Geometry check sheet. Reference: the model listing, model coordinates, mm. A direction names the side the tool comes from. Give positions to 0.01 mm unless a question says otherwise; leave off trailing zeros. Loops run counter-clockwise (first coordinate to the right, second up) from the corner with the lowest first, then second, coordinate; pieces in that order, holes last. Notation, with made-up numbers: (38, 20) -> (87, 20) arc R18 ccw to (87, 28) -> close; hole circle Ø9 at (59.5, 49.5). An arc over 180 degrees is marked (long way). One line per item, written item: value. Start each with the question number.
(1) Sectioned sample at A-A, the plane z = 0. Record the cut outline in (x, y) (3 decimals), then the cut area to 3 significant figures.
(2) Gauge pin test, flat ends, axial feed: pin 1 Ø4 at (y, z) = (6, -8.5) entering from +X; pin 2 Ø1.5 at (y, z) = (6.5, -4) entering from -X; pin 3 Ø5 at (x, y) = (10, 14.5) entering from +Z. Record the tip position at first contact, or that the pin passes through.
(3) Tool access check on faces 1 (the face through (0, 4, -2)), 2 (the face through (0, 17, 0)), 3 (the face through (2, 0, -10)). Record the directions out of +Z, -Z, +X, -X, +Y, -Y that give a thin tool (end or side, any length) a straight path to the whole face; none if there is none.
(4) Scan lines: line 1 along Z through (x, y) = (0, 17.4); line 2 along X through (y, z) = (10.25, 0); line 3 along Z through (x, y) = (2.5, 6.5). Record each from-to range of solid material in increasing order. Write a range as from..to.
(5) Sectioned sample at C-C, the plane x = 0. Record the cut outline in (y, z) (3 decimals), then the cut area to 3 significant figures.
(6) Sectioned sample at D-D, the plane x = 7.25. Record the cut outline in (y, z).
(7) Draft check along Z on faces 4 (the face through (-2.17, 3.94, -9.76)), 5 (the face through (2, 18, -10)), 6 (the face through (7.123, 8.874, -11.172)). Enter one of: pulls with the +Z half, pulls with the -Z half, needs draft (parallel to the pull), parting line crosses it, or undercut.
(8) Sectioned sample at B-B, the plane y = 3. Record the cut outline in (x, z), then the cut area to 3 significant figures.
from build123d import *

# Parameters (mm, degrees)
SKETCH1_R           = 13.25
BOSS_EXTRUDE1_DEPTH = 35
SKETCH7_R           = 10
CUT_EXTRUDE4_DEPTH  = 8
SKETCH10_R          = 3.485
BOSS_EXTRUDE3_DEPTH = 4
CUT_EXTRUDE5_DEPTH  = 8.75
SKETCH13_R          = 10
CUT_EXTRUDE6_DEPTH  = 18
SKETCH14_R          = 13.25
CUT_EXTRUDE7_DEPTH  = 17


with BuildPart() as part:
    # Sketch1 → Boss-Extrude1 (new body)
    with BuildSketch(Plane(origin=(0, 0, 0), x_dir=(1, 0, 0), z_dir=(0, 1, 0))):
        Circle(SKETCH1_R)
    extrude(amount=BOSS_EXTRUDE1_DEPTH)

    # Sketch7 → Cut-Extrude4 (cut)
    with BuildSketch(Plane.XZ):
        Circle(SKETCH7_R)
    extrude(amount=-CUT_EXTRUDE4_DEPTH, mode=Mode.SUBTRACT)

    # Sketch10 → Boss-Extrude3 (add)
    with BuildSketch(Plane.XZ.offset(-8)):
        Circle(SKETCH10_R)
    extrude(amount=BOSS_EXTRUDE3_DEPTH)

    # Sketch11 → Cut-Extrude5 (cut)
    with BuildSketch(Plane.XZ.offset(-4)):
        with BuildLine():
            Line((1.123990489, -1.161812868), (-1.123990489, -1.161812868))
            ThreePointArc((-1.123990489, -1.161812868), (0, 1.616528304), (1.123990489, -1.161812868))
        make_face()
    extrude(amount=-CUT_EXTRUDE5_DEPTH, mode=Mode.SUBTRACT)

    # Sketch13 → Cut-Extrude6 (cut)
    with BuildSketch(Plane(origin=(0, 35, 0), x_dir=(1, 0, 0), z_dir=(0, 1, 0))):
        Circle(SKETCH13_R)
    extrude(amount=-CUT_EXTRUDE6_DEPTH, mode=Mode.SUBTRACT)

    # Sketch14 → Cut-Extrude7 (cut)
    with BuildSketch(Plane(origin=(0, 35, 0), x_dir=(1, 0, 0), z_dir=(0, 1, 0))):
        Circle(SKETCH14_R)
    extrude(amount=-CUT_EXTRUDE7_DEPTH, mode=Mode.SUBTRACT)


solid = part.part
Calculated:
1. outline: (-13.25, 0) -> (-10, 0) -> (-10, 8) -> (-3.485, 8) -> (-3.485, 4) -> (-1.617, 4) -> (-1.617, 12.75) -> (1.617, 12.75) -> (1.617, 4) -> (3.485, 4) -> (3.485, 8) -> (10, 8) -> (10, 0) -> (13.25, 0) -> (13.25, 18) -> (10, 18) -> (10, 17) -> (-10, 17) -> (-10, 18) -> (-13.25, 18) -> close
1. area: 297 mm2
2. pin 1: stops at x = 11.55
2. pin 2: stops at x = -12.85
2. pin 3: stops at z = 10.92
3. face 1: -Y
3. face 2: +Y
3. face 3: +Z, -Z, +X, -X, -Y
4. line 1: z = -13.25..-10, 10..13.25
4. line 2: x = -13.25..-1.62, 1.62..13.25
4. line 3: z = -13.01..-9.68, -2.43..2.43, 9.68..13.01
5. outline: (0, -13.25) -> (18, -13.25) -> (18, -10) -> (17, -10) -> (17, 10) -> (18, 10) -> (18, 13.25) -> (0, 13.25) -> (0, 10) -> (8, 10) -> (8, 3.485) -> (4, 3.485) -> (4, 1.617) -> (12.75, 1.617) -> (12.75, -1.162) -> (4, -1.162) -> (4, -3.485) -> (8, -3.485) -> (8, -10) -> (0, -10) -> close
5. area: 301 mm2
6. outline: (0, -11.09) -> (18, -11.09) -> (18, -6.89) -> (17, -6.89) -> (17, 6.89) -> (18, 6.89) -> (18, 11.09) -> (0, 11.09) -> (0, 6.89) -> (8, 6.89) -> (8, -6.89) -> (0, -6.89) -> close
7. face 4: undercut
7. face 5: needs draft
7. face 6: parting line crosses it
8. outline: circle Ø26.5 at (0, 0); hole circle Ø20 at (0, 0)
8. area: 237 mm2
